The listing builds one solid part. Answer for the finished solid, in the listing's coordinates (mm). Round coordinates to 2 decimals unless told otherwise and drop trailing zeros. Write each loop counter-clockwise with the first axis right and the second up, starting at its lowest first coordinate (ties: lowest second). Pieces come first, ordered by that corner, then holes.
(1) Find the intervals of material crossed by probe 1 along Z at (x, y) = (144, -32); probe 2 along X at (y, z) = (-22.5, 468); probe 3 along Y at (x, z) = (13.5, 218), in increasing order.
(2) A cutting plane is placed at A-A, the plane z = 288.5. Give the vertices of the cut face in (x, y).
(3) Each of these flat-tipped pins is pushed along its axis until it touches: pin 1 Ø12 at (x, z) = (82.5, 232) entering from -Y; pin 2 Ø1.5 at (x, z) = (148, 1348.5) entering from -Y; pin 3 Ø18.5 at (x, z) = (32.5, 100) entering from -Y; pin 4 Ø10 at (x, z) = (36, 1533.5) entering from +Y. Where does it stop, or does it pass through?
from build123d import *

# Parameters (mm, degrees)
EXTRUDE_1_DEPTH             = 2000
EXTRUDE_2_DEPTH             = 5
HOLE_WIZARD_16_0_16_1_D     = 16
HOLE_WIZARD_16_0_16_2_D     = 16
HOLE_WIZARD_16_0_16_2_DEPTH = 5
HOLE_WIZARD_16_0_16_3_D     = 16
HOLE_WIZARD_16_0_16_3_DEPTH = 5


with BuildPart() as part:
    # Model → 凸台-拉伸1 (new body)
    with BuildSketch(Plane.XY):
        with BuildLine():
            Line((55, -147), (6, -147))
            Line((6, -147), (6, -150))
            Line((6, -150), (0, -150))
            Line((0, -150), (0, 0))
            Line((0, 0), (150, 0))
            Line((150, 0), (150, -6))
            Line((150, -6), (147, -6))
            Line((147, -6), (147, -55))
            Line((147, -55), (150, -58))
            Line((150, -58), (150, -65))
            Line((150, -65), (142, -65))
            Line((142, -65), (142, -6))
            Line((142, -6), (9, -6))
            ThreePointArc((9, -6), (6.878679656, -6.878679656), (6, -9))
            Line((6, -9), (6, -142))
            Line((6, -142), (65, -142))
            Line((65, -142), (65, -150))
            Line((65, -150), (58, -150))
            Line((58, -150), (55, -147))
        make_face()
    extrude(amount=EXTRUDE_1_DEPTH)

    # 草图2 → 凸台-拉伸2 (add)
    with BuildSketch(Plane.XY.offset(2000)):
        Polygon((65, -142), (65, -65), (142, -65), (142, -6), (6, -6), (6, -142), align=None)
    extrude_2 = extrude(amount=-EXTRUDE_2_DEPTH)

    # 镜向1: 凸台-拉伸2 across plane
    add(extrude_2.mirror(Plane.XY.offset(1000)))

    # Ø16.0 (16) 直径孔1 (through all)
    with Locations(Plane.XY.offset(2000)):
        with Locations((100, -32.5), (32.5, -100)):
            Hole(HOLE_WIZARD_16_0_16_1_D / 2)

    # Ø16.0 (16) 直径孔2
    with Locations(Plane(origin=(147, 0, 0), x_dir=(0, 0, -1), z_dir=(1, 0, 0))):
        with Locations((-1950, -32.5), (-1900, -32.5), (-50, -32.5), (-100, -32.5)):
            Hole(HOLE_WIZARD_16_0_16_2_D / 2, depth=HOLE_WIZARD_16_0_16_2_DEPTH)

    # Ø16.0 (16) 直径孔3
    with Locations(Plane(origin=(0, -147, 0), x_dir=(-1, 0, 0), z_dir=(0, -1, 0))):
        with Locations((-32.5, -1950), (-32.5, -1900), (-32.5, -50), (-32.5, -100)):
            Hole(HOLE_WIZARD_16_0_16_3_D / 2, depth=HOLE_WIZARD_16_0_16_3_DEPTH)


solid = part.part
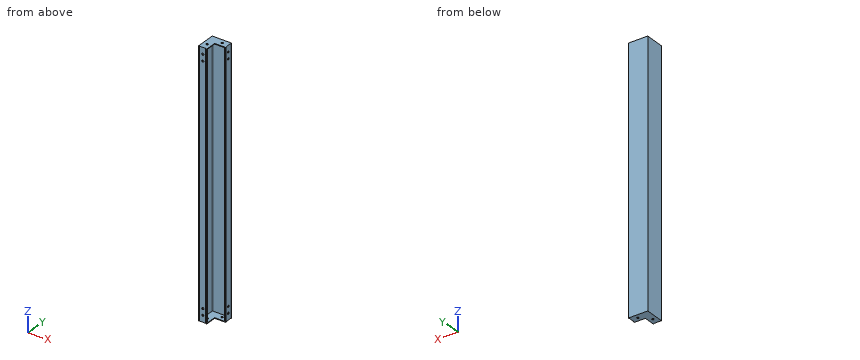
Solutions:
1. probe 1: z = 0 to 42.02, 57.98 to 92.02, 107.98 to 1892.02, 1907.98 to 1942.02, 1957.98 to 2000
1. probe 2: x = 0 to 6, 142 to 147
1. probe 3: y = -147 to -142, -6 to 0
2. outline: (0, -150) - (6, -150) - (6, -147) - (55, -147) - (58, -150) - (65, -150) - (65, -142) - (6, -142) - (6, -9) arc R3 cw to (9, -6) - (142, -6) - (142, -65) - (150, -65) - (150, -58) - (147, -55) - (147, -6) - (150, -6) - (150, 0) - (0, 0) - close
3. pin 1: stops at y = -6
3. pin 2: stops at y = -65
3. pin 3: stops at y = -147
3. pin 4: stops at y = 0
